Here's how the part is built. I have some questions about the finished solid (model axes, mm). Face numbers are marked on the shaded views. A direction names the side the tool comes from. Round coordinates to 2 decimals unless told otherwise and drop trailing zeros. Order: outer loops, then holes, each group sorted by start corner. A loop starts at its lowest first (then second) coordinate and runs counter-clockwise, first axis right, second up.
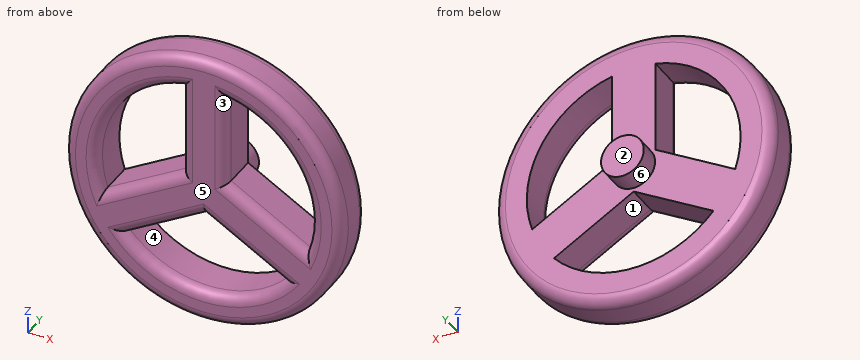
```python
from build123d import *

# Parameters (mm, degrees)
F0_R     = 10
F1_DEPTH = 10
F3_R     = 65
F4_DEPTH = 20
F6_DEPTH = 20
F7_R     = 5


with BuildPart() as f1:
    # F0 (on Front) → F1 (new body)
    with BuildSketch(Plane.XZ):
        Circle(F0_R)
    extrude(amount=F1_DEPTH)

    # F3 (on offset) → F4 (join, through all)
    with BuildSketch(Plane.XZ.offset(30)):
        Circle(F3_R)
    extrude(amount=-F4_DEPTH)

    # F5 (on face) → F6 (cut, through all)
    with BuildSketch(Plane.XZ.offset(30)):
        with BuildLine():
            Line((-47.487018, -15.651937), (-10.188534, 5.882353))
            Line((-10.188534, 5.882353), (-10.188534, 48.950932))
            ThreePointArc((-10.188534, 48.950932), (-43.30127, 25), (-47.487018, -15.651937))
        make_face()
        with BuildLine():
            Line((10.188534, 48.950932), (10.188534, 5.882353))
            Line((10.188534, 5.882353), (47.487018, -15.651937))
            ThreePointArc((47.487018, -15.651937), (43.30127, 25), (10.188534, 48.950932))
        make_face()
        with BuildLine():
            Line((0, -11.764706), (-37.298484, -33.298996))
            ThreePointArc((-37.298484, -33.298996), (0, -50), (37.298484, -33.298996))
            Line((37.298484, -33.298996), (0, -11.764706))
        make_face()
    extrude(amount=-F6_DEPTH, mode=Mode.SUBTRACT)

    # F7
    f7_edges = [f1.edges().sort_by_distance(p)[0] for p in [
        (-65, -30, 0),
        (18.649242, -30, -22.531851),
        (-18.649242, -30, -22.531851),
        (0, -30, -50),
        (-28.837776, -30, -4.884792),
        (-10.188534, -30, 27.416643),
        (-43.30127, -30, 25),
        (10.188534, -30, 27.416643),
        (28.837776, -30, -4.884792),
        (43.30127, -30, 25),
        (65, -20, 0),
        (-65, -10, 0),
    ]]
    fillet(f7_edges, radius=F7_R)


solid = f1.part
```
1) I'm going to push flat-ended pins straight in: pin 1 (12 mm diameter, centred on x = -36.5, y = -9.5, fed in from -Z); pin 2 (12 mm diameter, centred on x = -13, y = -26, fed in from +Z); pin 3 (10 mm diameter, centred on x = -33, z = 3.5, fed in from +Y); pin 4 (16.5 mm diameter, centred on y = -16, z = 37, fed in from -X). Where does each tip first touch, or does it pass through?
2) We'd pull the mould along Z, two halves only. Please class the marked faces 4, 5 and 6: +Z half, -Z half, draft (parallel to the pull), parting line (faces both ways), or undercut.
3) For the marked faces 1, 2 and 3, which set-ups out of +Z, -Z, +X, -X, +Y, -Y let a thin tool reach every point of the face, with its end or its side?
4) If we section it at C-C (y = -4.5): Write out the boundary of the cut face in (x, z), plus the area to 3 significant figures.
5) If we section it at A-A (x = -14.5): Give the number of separate pieces and of enclosed holes in the cut face, plus the area to 3 significant figures.
6) I need wall thicknesses on line 1 (X direction, y = -18, z = 1); line 2 (X direction, y = -19, z = 19); line 3 (Z direction, x = -28, y = -21.5). Which ranges of each line are inside material? Lowest first, please.
Solutions:
1. pin 1: stops at z = -56.32
1. pin 2: stops at z = 64.61
1. pin 3: passes through
1. pin 4: stops at x = -58.3
2. face 4: undercut
2. face 5: draft
2. face 6: parting line
3. face 1: +Y, -Y
3. face 2: +Z, -Z, +X, -X, +Y
3. face 3: -Y
4. outline: circle Ø20 at (0, 0)
4. area: 314 mm2
5. separate pieces: 3
5. enclosed holes: 0
5. area: 1,050 mm2
6. line 1: x = -64.99 to -49.99, -18.65 to 18.65, 49.99 to 64.99
6. line 2: x = -62.16 to -46.25, -10.19 to 10.19, 46.25 to 62.16
6. line 3: z = -58.66 to -41.42, -27.93 to -4.4, 41.42 to 58.66
